Verification items for this drawing (mm, ordinates from the low corner). A direction names the side the tool comes from. Round coordinates to 2 decimals unless told otherwise and drop trailing zeros. Write each loop counter-clockwise with the first axis right and the second up, starting at its lowest first coordinate (ties: lowest second). Pieces come first, ordered by that corner, then holes. Notation, with made-up numbers: (34, 23) -> (66, 23) arc R16 cw to (66, 33) -> close; hole circle Ø7 at (38.5, -4). An arc over 180 degrees is marked (long way). One line per question, with ' | ' between items.
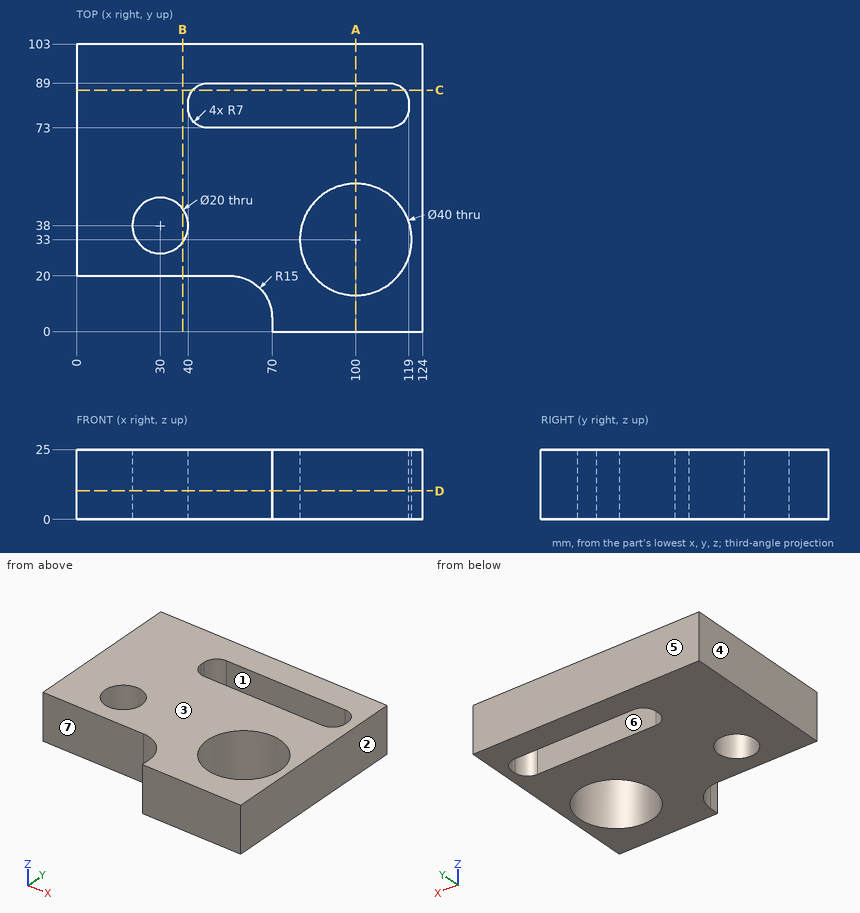
(1) Sectioned sample at D-D on z = 10.25. Record the cut outline in (x, y), then the cut area to 3 significant figures.
Resolved:
outline: (0, 20) -> (55, 20) arc R15 cw to (70, 5) -> (70, 0) -> (124, 0) -> (124, 103) -> (0, 103) -> close; hole circle Ø20 at (30, 38); hole (40, 80) arc R7 ccw to (47, 73) -> (112, 73) arc R7 ccw to (119, 80) -> (119, 82) arc R7 ccw to (112, 89) -> (47, 89) arc R7 ccw to (40, 82) -> close; hole circle Ø40 at (100, 33) | area: 8,630 mm2
(2) Sectioned sample at B-B on x = 38. Record the cut outline in (y, z).
Resolved:
outline: (20, 0) -> (32, 0) -> (32, 25) -> (20, 25) -> close; (44, 0) -> (103, 0) -> (103, 25) -> (44, 25) -> close
(3) Sectioned sample at C-C on y = 86.5. Record the cut outline in (x, z).
Resolved:
outline: (0, 0) -> (41.64, 0) -> (41.64, 25) -> (0, 25) -> close; (117.36, 0) -> (124, 0) -> (124, 25) -> (117.36, 25) -> close
(4) Sectioned sample at A-A on x = 100. Record the cut outline in (y, z), then the cut area to 4 significant figures.
Resolved:
outline: (0, 0) -> (13, 0) -> (13, 25) -> (0, 25) -> close; (53, 0) -> (73, 0) -> (73, 25) -> (53, 25) -> close; (89, 0) -> (103, 0) -> (103, 25) -> (89, 25) -> close | area: 1,175 mm2
(5) Material ranges on line 1 (Y direction, x = 100, z = 5.75); line 2 (Y direction, x = 30, z = 15.25); line 3 (Y direction, x = 76, z = 5.75), recorded low to high.
Resolved:
line 1: y = 0 to 13, 53 to 73, 89 to 103 | line 2: y = 20 to 28, 48 to 103 | line 3: y = 0 to 73, 89 to 103
(6) Draft check along X on the marked faces 1, 2, 3 and 4. Enter one of: +X half, -X half, draft (parallel to the pull), parting line (faces both ways), or undercut.
Resolved:
face 1: undercut | face 2: +X half | face 3: draft | face 4: -X half
(7) Go/stop test with flat-tipped pins: pin 1 (12.5 mm diameter, centred on x = 15.5, z = 13, fed in from -Y); pin 2 (5.5 mm diameter, centred on y = 3.5, z = 9, fed in from -X); pin 3 (8 mm diameter, centred on x = 88, y = 25.5, fed in from -Z); pin 4 (8 mm diameter, centred on x = 61.5, z = 17, fed in from -Y). Record where each tip stops, or that it passes through.
Resolved:
pin 1: stops at y = 20 | pin 2: stops at x = 69.95 | pin 3: passes through | pin 4: stops at y = 15.71
(8) Access from +Z, -Z, +X, -X, +Y, -Y to the whole of each face (thin tool, end or side, straight path). Record for the marked faces 5, 6 and 7.
Resolved:
face 5: +Z, -Z, +X, -X, +Y | face 6: +Z, -Z | face 7: +Z, -Z, -X, -Y
